from build123d import *

# Parameters (mm, degrees)
SKETCH1_W           = 112
SKETCH1_H           = 215
BOSS_EXTRUDE1_DEPTH = 2
SKETCH2_W           = 29.333333333
SKETCH2_H           = 47.75
SKETCH2_W_2         = 29.333333334
CUT_EXTRUDE1_DEPTH  = 1.5
CUT_EXTRUDE2_DEPTH  = 122.228090804
SKETCH4_R           = 1.35
CUT_EXTRUDE3_DEPTH  = 122.228090804
FILLET1_R           = 3.175
FILLET2_R           = 3.175
CUT_EXTRUDE4_DEPTH  = 122.228090804
FILLET3_R           = 0.3


with BuildPart() as part:
    # Sketch1 → Boss-Extrude1 (new body)
    with BuildSketch(Plane(origin=(0, 0, 0), x_dir=(1, 0, 0), z_dir=(0, 1, 0))):
        Rectangle(SKETCH1_W, SKETCH1_H)
    extrude(amount=BOSS_EXTRUDE1_DEPTH)

    # Sketch2 → Cut-Extrude1 (cut)
    with BuildSketch(Plane(origin=(0, 2, 0), x_dir=(1, 0, 0), z_dir=(0, 1, 0))):
        with Locations((-32.333333334, 77.625)):
            Rectangle(SKETCH2_W, SKETCH2_H)
        with Locations((-32.333333334, 25.875)):
            Rectangle(SKETCH2_W, SKETCH2_H)
        with Locations((0, 77.625)):
            Rectangle(SKETCH2_W_2, SKETCH2_H)
        with Locations((0, 25.875)):
            Rectangle(SKETCH2_W_2, SKETCH2_H)
        with Locations((-32.333333334, -25.875)):
            Rectangle(SKETCH2_W, SKETCH2_H)
        with Locations((32.333333334, 77.625)):
            Rectangle(SKETCH2_W, SKETCH2_H)
        with Locations((32.333333334, 25.875)):
            Rectangle(SKETCH2_W, SKETCH2_H)
        with Locations((0, -25.875)):
            Rectangle(SKETCH2_W_2, SKETCH2_H)
        with Locations((32.333333334, -25.875)):
            Rectangle(SKETCH2_W, SKETCH2_H)
        with Locations((32.333333334, -77.625)):
            Rectangle(SKETCH2_W, SKETCH2_H)
        with Locations((0, -77.625)):
            Rectangle(SKETCH2_W_2, SKETCH2_H)
        with Locations((-32.333333334, -77.625)):
            Rectangle(SKETCH2_W, SKETCH2_H)
    extrude(amount=-CUT_EXTRUDE1_DEPTH, mode=Mode.SUBTRACT)

    # Sketch3 → Cut-Extrude2 (cut, through all)
    with BuildSketch(Plane(origin=(0, 2, 0), x_dir=(1, 0, 0), z_dir=(0, 1, 0))):
        Polygon((-56, 107.5), (-53.5, 107.5), (-56, 97.5), align=None)
        Polygon((56, 107.5), (53.5, 107.5), (56, 97.5), align=None)
        Polygon((56, -107.5), (56, -97.5), (53.5, -107.5), align=None)
        Polygon((-56, -107.5), (-56, -97.5), (-53.5, -107.5), align=None)
    extrude(amount=-CUT_EXTRUDE2_DEPTH, mode=Mode.SUBTRACT)

    # Sketch4 → Cut-Extrude3 (cut, through all)
    with BuildSketch(Plane(origin=(0, 2, 0), x_dir=(1, 0, 0), z_dir=(0, 1, 0))):
        with Locations(Location((-50, 104.5, 0), (0, 0, 270))):
            Circle(SKETCH4_R)
        with Locations(Location((-50, -104.5, 0), (0, 0, 270))):
            Circle(SKETCH4_R)
        with Locations(Location((50, -104.5, 0), (0, 0, 90))):
            Circle(SKETCH4_R)
        with Locations(Location((50, -25, 0), (0, 0, 90))):
            Circle(SKETCH4_R)
        with Locations(Location((50, 25, 0), (0, 0, 90))):
            Circle(SKETCH4_R)
        with Locations(Location((50, 104.5, 0), (0, 0, 90))):
            Circle(SKETCH4_R)
        with Locations(Location((-50, 77.5, 0), (0, 0, 270))):
            Circle(SKETCH4_R)
        with Locations(Location((-50, 25, 0), (0, 0, 270))):
            Circle(SKETCH4_R)
        with Locations(Location((-50, -25, 0), (0, 0, 270))):
            Circle(SKETCH4_R)
        with Locations(Location((-50, -77.5, 0), (0, 0, 270))):
            Circle(SKETCH4_R)
        with Locations(Location((50, -77.5, 0), (0, 0, 270))):
            Circle(SKETCH4_R)
        with Locations(Location((50, 77.5, 0), (0, 0, 270))):
            Circle(SKETCH4_R)
    extrude(amount=-CUT_EXTRUDE3_DEPTH, mode=Mode.SUBTRACT)

    # Fillet1
    fillet1_edges = [part.edges().sort_by_distance(p)[0] for p in [
        (-17.666666667, 1.25, -101.5),
        (-17.666666667, 1.25, -53.75),
        (-47, 1.25, -53.75),
        (-47, 1.25, -101.5),
        (-47, 1.25, 101.5),
        (-47, 1.25, 53.75),
        (-17.666666667, 1.25, 101.5),
        (14.666666667, 1.25, 53.75),
        (14.666666667, 1.25, 101.5),
        (-14.666666667, 1.25, 101.5),
        (-14.666666667, 1.25, 53.75),
        (47, 1.25, 53.75),
        (47, 1.25, 101.5),
        (17.666666667, 1.25, 101.5),
        (17.666666667, 1.25, 53.75),
        (17.666666667, 1.25, -53.75),
        (17.666666667, 1.25, -101.5),
        (47, 1.25, -101.5),
        (47, 1.25, -53.75),
        (-14.666666667, 1.25, -2),
        (-14.666666667, 1.25, -49.75),
        (14.666666667, 1.25, -49.75),
        (14.666666667, 1.25, -2),
        (-14.666666667, 1.25, -53.75),
        (-14.666666667, 1.25, -101.5),
        (14.666666667, 1.25, -101.5),
        (14.666666667, 1.25, -53.75),
        (-47, 1.25, -2),
        (-47, 1.25, -49.75),
        (-17.666666667, 1.25, -2),
        (47, 1.25, 2),
        (47, 1.25, 49.75),
        (17.666666667, 1.25, 49.75),
        (17.666666667, 1.25, 2),
        (14.666666667, 1.25, 2),
        (14.666666667, 1.25, 49.75),
        (-14.666666667, 1.25, 49.75),
        (-14.666666667, 1.25, 2),
        (-17.666666667, 1.25, 49.75),
        (-47, 1.25, 49.75),
        (-47, 1.25, 2),
        (17.666666667, 1.25, -2),
        (17.666666667, 1.25, -49.75),
        (47, 1.25, -49.75),
        (47, 1.25, -2),
    ]]
    fillet(fillet1_edges, radius=FILLET1_R)

    # Fillet2
    fillet2_edges = [part.edges().sort_by_distance(p)[0] for p in [
        (-17.666666667, 1.25, 53.75),
        (-17.666666667, 1.25, -49.75),
        (-17.666666667, 1.25, 2),
    ]]
    fillet(fillet2_edges, radius=FILLET2_R)

    # Sketch9 → Cut-Extrude4 (cut, through all)
    with BuildSketch(Plane(origin=(0, 2, 0), x_dir=(1, 0, 0), z_dir=(0, 1, 0))):
        with BuildLine():
            Line((-56, 66.961249469), (-55.251016984, 66.929117979))
            ThreePointArc((-55.251016984, 66.929117979), (-54.10373807, 66.364425295), (-53.744982789, 65.137061706))
            Line((-53.744982789, 65.137061706), (-54.112689456, 62.327568098))
            ThreePointArc((-54.112689456, 62.327568098), (-54.685065741, 61.302017235), (-55.805706914, 60.950545264))
            ThreePointArc((-55.805706914, 60.950545264), (-56.544843899, 60.751892413), (-56.927023895, 60.088774861))
            Line((-56.927023895, 60.088774861), (-57.5, 60.088774861))
            Line((-57.5, 60.088774861), (-57.5, 66.961249469))
            Line((-57.5, 66.961249469), (-56, 66.961249469))
        make_face()
        with BuildLine():
            Line((57.5, 66.961249469), (57.5, 60.088774861))
            Line((57.5, 60.088774861), (56.927023895, 60.088774861))
            ThreePointArc((56.927023895, 60.088774861), (56.544843899, 60.751892413), (55.805706914, 60.950545264))
            ThreePointArc((55.805706914, 60.950545264), (54.685065741, 61.302017235), (54.112689456, 62.327568098))
            Line((54.112689456, 62.327568098), (53.744982789, 65.137061706))
            ThreePointArc((53.744982789, 65.137061706), (54.10373807, 66.364425295), (55.251016984, 66.929117979))
            Line((55.251016984, 66.929117979), (56, 66.961249469))
            Line((56, 66.961249469), (57.5, 66.961249469))
        make_face()
    extrude(amount=-CUT_EXTRUDE4_DEPTH, mode=Mode.SUBTRACT)

    # Fillet3
    fillet3_edges = [part.edges().sort_by_distance(p)[0] for p in [
        (56, 1, -66.961249469),
        (56, 1, -60.956917999),
        (-56, 1, -60.956917999),
        (-56, 1, -66.961249469),
    ]]
    fillet(fillet3_edges, radius=FILLET3_R)


solid = part.part
Can you work these out from the model? Positions are in its coordinate system, mm. A direction names the side the tool comes from. Give positions to 0.01 mm unless a question says otherwise; leave off trailing zeros. Write each loop counter-clockwise with the first axis right and the second up, starting at its lowest first coordinate (ties: lowest second). Pieces come first, ordered by that corner, then holes. Notation, with made-up numbers: (82.5, 42) -> (115.5, 42) arc R21 cw to (115.5, 73) -> close; hole circle Ø1 at (43.25, 6.25). An arc over 180 degrees is marked (long way). Answer as a JSON object with one key per item and string values. Group by question number.
Item 1: We'd pull the mould along Z, two halves only. Please class faces 1 (the face through (-1, 0, -2)), 2 (the face through (32, 0.5, 26)), 3 (the face through (-33, 0.5, -26)): +Z half, -Z half, draft (parallel to the pull), parting line (faces both ways), or undercut.
Item 2: For faces 4 (the face through (-33, 0.5, 77)), 5 (the face through (8, 2, -1)), which set-ups out of +Z, -Z, +X, -X, +Y, -Y let a thin tool reach every point of the face, with its end or its side?
Item 3: Please list where these lines run through material, in increasing order: line 1 (X direction, y = 0.7, z = 25); line 2 (X direction, y = 1, z = -36); line 3 (Z direction, x = -41, y = 0.8). Write a range as [from, to].
Item 4: Suppose I cut it at B-B (x = 26). Please give me the cut outline in (y, z), plus the area to 4 significant figures.
Item 5: Suppose I cut it at A-A (z = 63). Please give me the cut outline in (x, y).
Item 6: I'm going to push flat-ended pins straight in: P1, Ø23.5, axis at x = 32, z = 27, coming from the +Y side; P2, Ø3, axis at x = -19.5, z = -45, coming from the -Y side. Where does each tip first touch, or does it pass through?
Findings:
{
 "1": {"face 1": "draft", "face 2": "undercut", "face 3": "undercut"},
 "2": {"face 4": "+Y", "face 5": "+Z, -Z, +X, -X, +Y"},
 "3": {"line 1": "x = [-56, -51.35], [-48.65, -47], [-17.67, -14.67], [14.67, 17.67], [47, 48.65], [51.35, 56]", "line 2": "x = [-56, -47], [-17.67, -14.67], [14.67, 17.67], [47, 56]", "line 3": "z = [-107.5, -101.5], [-53.75, -49.75], [-2, 2], [49.75, 53.75], [101.5, 107.5]"},
 "4": {"outline": "(0, -107.5) -> (2, -107.5) -> (2, -101.5) -> (0.5, -101.5) -> (0.5, -53.75) -> (2, -53.75) -> (2, -49.75) -> (0.5, -49.75) -> (0.5, -2) -> (2, -2) -> (2, 2) -> (0.5, 2) -> (0.5, 49.75) -> (2, 49.75) -> (2, 53.75) -> (0.5, 53.75) -> (0.5, 101.5) -> (2, 101.5) -> (2, 107.5) -> (0, 107.5) -> close", "area": "143.5 mm²"},
 "5": {"outline": "(-56, 0) -> (56, 0) -> (56, 2) -> (47, 2) -> (47, 0.5) -> (17.67, 0.5) -> (17.67, 2) -> (14.67, 2) -> (14.67, 0.5) -> (-14.67, 0.5) -> (-14.67, 2) -> (-17.67, 2) -> (-17.67, 0.5) -> (-47, 0.5) -> (-47, 2) -> (-56, 2) -> close"},
 "6": {"P1": "stops at y = 0.5", "P2": "stops at y = 0"}
}
